Autodesk Inventor part; units mm, degrees
ref_plane "YZ Plane" through (0, 0, 0) normal (1, 0, 0) x (0, 1, 0)
ref_plane "XZ Plane" through (0, 0, 0) normal (0, 1, 0) x (-1, 0, 0)
ref_plane "XY Plane" through (0, 0, 0) normal (0, 0, 1) x (1, 0, 0)
sketch "Skizze2" plane through (0, 0, 0) normal (0, 0, 1) x (1, 0, 0)
  line L0 (-44.5, 0) -> (44.5, 0)
  line L1 (44.5, 0) -> (44.5, 67)
  line L2 (44.5, 67) -> (-44.5, 67)
  line L3 (-44.5, 67) -> (-44.5, 0)
  point P0 (0, 0)
  point P1 (0, 0)
  dimension "d0" = 89
  dimension "d1" = 67
extrude "Extrusion1" add sketch "Skizze2" along normal blind 36
shell "Wandung1" thickness 1.5 removed faces 1 at (-14.8333, 44.6667, 36)
sketch "Skizze3" plane through (44.5, 0, 0) normal (1, 0, 0) x (0, 0, -1)
  circle A0 centre (-14, 32) radius 11
  line L0 (0, 0) -> (0, 67)
  line L1 (0, 67) -> (-36, 67)
  dimension "d5" = 22
  dimension "d6" = 14
  dimension "d7" = 35
extrude "Extrusion2" cut sketch "Skizze3" against normal up to surface (1.5 mm away)
fillet "Rundung1" radius 1 12 edges at (44.5, 67, 18) (44.5, 0, 18) (-44.5, 0, 18) (-44.5, 67, 18) (-43, 65.5, 18.75) (43, 65.5, 18.75) (43, 1.5, 18.75) (-43, 1.5, 18.75) (-43, 33.5, 1.5) (0, 1.5, 1.5) (43, 33.5, 1.5) (0, 65.5, 1.5)
properties part number "102 part 1" material "Aluminum 6061, geschweißt"
For this review, take the finished solid that the model builds, in its own axes (mm). A direction names the side the tool comes from. Coordinates: 2 decimals unless noted, no trailing zeros. Order: outer loops, then holes, each group sorted by start corner. A loop starts at its lowest first (then second) coordinate and runs counter-clockwise, first axis right, second up. Notation, with made-up numbers: (30.25, 34) - (34.25, 34) arc R18 ccw to (34.25, 58) - close; hole circle Ø6 at (-11, 27). An arc over 180 degrees is marked (long way). Answer as CSV lines item,"result". Start each with the question number.
1) Add section C-C (z = 14). State the section outline as (x, y) points, then the cut area to 3 significant figures.
2) Add section B-B (z = 31.5). State the section outline as (x, y) points, then the cut area to 3 significant figures.
3) Machinability: for faces 1 (the flat face through (44.5, 33, 26)), 2 (the flat face through (1, 65.5, 19)), which of the approach directions +Z, -Z, +X, -X, +Y, -Y give a long, thin tool a straight path to every point of the face, cutting with its end or side? Answer none if there is none.
4) Insertion check: P1, Ø4, axis at x = 10.5, y = 60, coming from the +Z side. The pin has a flat end and moves straight along its axis. Give the tip position at first contact, or say it passes through.
5) Draft analysis for pull direction Z (two halves, no side actions). For faces 3 (the flat face through (-44.5, 34, 18)), 4 (the cylindrical face through (43.76, 22.241, 8.924)), 5 (the flat face through (-1, 34, 1.5)), 6 (the flat face through (-1, 34, 0)), state which applies: +Z half, -Z half, draft (parallel to the pull), parting line (faces both ways), or undercut.
6) To check wall thickness, follow line 1 along Y through (x, z) = (-15.5, 10.5); line 2 along X through (y, z) = (28.5, 3); line 3 along Y through (x, z) = (43.45, 14). State the ranges of each line that lie inside material, in increasing order. Write a range as [from, to].
7) Add section D-D (x = -33.5). State the section outline as (y, z) points.
8) Add section A-A (y = 32). State the section outline as (x, z) points, then the cut area to 3 significant figures.
Result:
1,outline,"(-44.5, 1) arc R1 ccw to (-43.5, 0) - (43.5, 0) arc R1 ccw to (44.5, 1) - (44.5, 21) - (43, 21) - (43, 2.5) arc R1 cw to (42, 1.5) - (-42, 1.5) arc R1 cw to (-43, 2.5) - (-43, 64.5) arc R1 cw to (-42, 65.5) - (42, 65.5) arc R1 cw to (43, 64.5) - (43, 43) - (44.5, 43) - (44.5, 66) arc R1 ccw to (43.5, 67) - (-43.5, 67) arc R1 ccw to (-44.5, 66) - close"
1,area,"426 mm^2"
2,outline,"(-44.5, 1) arc R1 ccw to (-43.5, 0) - (43.5, 0) arc R1 ccw to (44.5, 1) - (44.5, 66) arc R1 ccw to (43.5, 67) - (-43.5, 67) arc R1 ccw to (-44.5, 66) - close; hole (-43, 2.5) arc R1 ccw to (-42, 1.5) - (42, 1.5) arc R1 ccw to (43, 2.5) - (43, 64.5) arc R1 ccw to (42, 65.5) - (-42, 65.5) arc R1 ccw to (-43, 64.5) - close"
2,area,"459 mm^2"
3,face 1,"+Z, -Z, +X, +Y, -Y"
3,face 2,"+Z"
4,P1,"z = 1.5"
5,face 3,"draft"
5,face 4,"undercut"
5,face 5,"+Z half"
5,face 6,"-Z half"
6,line 1,"[0, 1.5], [65.5, 67]"
6,line 2,"[-44.5, -43], [43, 44.5]"
6,line 3,"[0, 21], [43, 67]"
7,outline,"(0, 0) - (67, 0) - (67, 36) - (65.5, 36) - (65.5, 2.5) arc R1 cw to (64.5, 1.5) - (2.5, 1.5) arc R1 cw to (1.5, 2.5) - (1.5, 36) - (0, 36) - close"
8,outline,"(-44.5, 0) - (44.5, 0) - (44.5, 3) - (43, 3) - (43, 2.5) arc R1 cw to (42, 1.5) - (-42, 1.5) arc R1 cw to (-43, 2.5) - (-43, 36) - (-44.5, 36) - close; (43, 25) - (44.5, 25) - (44.5, 36) - (43, 36) - close"
8,area,"204 mm^2"
